The listing builds one solid part. Answer for the finished solid, in the listing's coordinates (mm). A direction names the side the tool comes from. Give positions to 0.01 mm unless a question says otherwise; leave off trailing zeros. Write each loop counter-clockwise with the first axis right and the second up, starting at its lowest first coordinate (ties: lowest second). Pieces come first, ordered by that corner, then holes. Notation, with made-up numbers: M 2,38 L 60,38 A23 ccw 60,73 Z; hole C 15.5,35.25 d4. An arc over 180 degrees is marked long. Answer as a JSON object with one key per item and string values.
```python
from build123d import *

# Parameters (mm, degrees)
BOSS_EXTRUDE1_DEPTH = 12
SKETCH2_W           = 130
SKETCH2_H           = 45
SKETCH2_W_2         = 170
SKETCH2_H_2         = 15
CUT_EXTRUDE1_DEPTH  = 609.394608786
CHAMFER1_SIZE       = 12
CUT_EXTRUDE2_START  = -10
SKETCH3_R           = 2.5
CUT_EXTRUDE2_DEPTH  = 150
CUT_EXTRUDE3_START  = 370
SKETCH3_2_R         = 2.5
CUT_EXTRUDE3_DEPTH  = 150


with BuildPart() as part:
    # Sketch1 → Boss-Extrude1 (new body)
    with BuildSketch(Plane.XY):
        with BuildLine():
            Line((0, 0), (0, -10))
            Line((0, -10), (40, -10))
            ThreePointArc((40, -10), (48.819660113, -2.639320225), (60, 0))
            Line((60, 0), (540, 0))
            ThreePointArc((540, 0), (551.180339887, -2.639320225), (560, -10))
            Line((560, -10), (600, -10))
            Line((600, -10), (600, 0))
            Line((600, 0), (600, 100))
            Line((600, 100), (0, 100))
            Line((0, 100), (0, 0))
        make_face()
    extrude(amount=BOSS_EXTRUDE1_DEPTH)

    # Sketch2 → Cut-Extrude1 (cut, through all)
    with BuildSketch(Plane.XY.offset(12)):
        with Locations((110, 42.5)):
            Rectangle(SKETCH2_W, SKETCH2_H)
        with Locations((300, 42.5)):
            Rectangle(SKETCH2_W_2, SKETCH2_H_2)
        with Locations((490, 42.5)):
            Rectangle(SKETCH2_W, SKETCH2_H)
    extrude(amount=-CUT_EXTRUDE1_DEPTH, mode=Mode.SUBTRACT)

    # Chamfer1
    chamfer1_edges = [part.edges().sort_by_distance(p)[0] for p in [
        (600, 45, 12),
        (300, 100, 12),
        (0, 45, 12),
    ]]
    chamfer(chamfer1_edges, length=CHAMFER1_SIZE - 0.0001)  # a hair under: the kernel refuses the full size

    # Sketch3 → Cut-Extrude2 (cut)
    with BuildSketch(Plane(origin=(45, 0, 0), x_dir=(0, 0, -1), z_dir=(1, 0, 0)).offset(CUT_EXTRUDE2_START)):
        with Locations((-4, 25)):
            Circle(SKETCH3_R)
    extrude(amount=CUT_EXTRUDE2_DEPTH, mode=Mode.SUBTRACT)

    # Sketch3<2> → Cut-Extrude3 (cut)
    with BuildSketch(Plane(origin=(45, 0, 0), x_dir=(0, 0, -1), z_dir=(1, 0, 0)).offset(CUT_EXTRUDE3_START)):
        with Locations((-4, 25)):
            Circle(SKETCH3_2_R)
    extrude(amount=CUT_EXTRUDE3_DEPTH, mode=Mode.SUBTRACT)


solid = part.part
```
1. A cutting plane is placed at C-C, the plane z = 8.75. Give the vertices of the cut face in (x, y).
Verdict:
{"outline": "M 8.75,-10 L 40,-10 A25 cw 60,0 L 540,0 A25 cw 560,-10 L 591.25,-10 L 591.25,91.25 L 8.75,91.25 Z; hole M 45,20 L 175,20 L 175,65 L 45,65 Z; hole M 215,35 L 385,35 L 385,50 L 215,50 Z; hole M 425,20 L 555,20 L 555,65 L 425,65 Z"}
2. Flat-ended cylindrical pins translate along their axes: pin 1 (1.5 mm diameter, centred on y = 24, z = 3, fed in from -X); pin 2 (6.5 mm diameter, centred on y = 25, z = 4, fed in from +X); pin 3 (4 mm diameter, centred on x = 286.5, z = 5.5, fed in from -Y). Find the tip coordinate at first contact, or state that the pin passes through.
Verdict:
{"pin 1": "stops at x = 2.25", "pin 2": "stops at x = 599.25", "pin 3": "stops at y = 0"}
3. A cutting plane is placed at A-A, the plane y = 42. Count the separate pieces of the cut face and the enclosed holes in it, plus the area to 3 significant figures.
Verdict:
{"separate pieces": "4", "enclosed holes": "0", "area": "1,900 mm2"}
4. The mould has two halves that part along Y. Classify faces 4 (the flat face through (304, 94, 6)), 5 (the flat face through (109, 20, 6)), 6 (the cylindrical face through (551.035, -2.567, 5.916)): released by +Y, released by -Y, zero draft, split by the parting line, or undercut.
Verdict:
{"face 4": "released by +Y", "face 5": "undercut", "face 6": "released by -Y"}
5. Consider line 1 along Z through (x, y) = (40.25, 25); line 2 along X through (y, z) = (43.5, 7.5); line 3 along X through (y, z) = (63, 1.5). Determine where each line is inside the solid, lowest interval first.
Verdict:
{"line 1": "z = 0 to 1.5, 6.5 to 12", "line 2": "x = 7.5 to 45, 175 to 215, 385 to 425, 555 to 592.5", "line 3": "x = 1.5 to 45, 175 to 425, 555 to 598.5"}
6. For faces 1 (the cylindrical face through (48.7, -2.7, 5.9)), 2 (the flat face through (45, 42, 6)), 3 (the flat face through (296, 51, 12)), determine the directions among +Z, -Z, +X, -X, +Y, -Y from which every point of the face is accessible in a straight line to the end or side of a thin tool.
Verdict:
{"face 1": "+Z, -Z, -Y", "face 2": "+Z, -Z", "face 3": "+Z, +X, -X, +Y, -Y"}
